```python
from build123d import *

# Parameters (mm, degrees)
SKETCH1_W                      = 50
SKETCH1_H                      = 100
SKETCH1_R                      = 15.2
SKETCH1_R_2                    = 2
BOSS_EXTRUDE1_DEPTH            = 33
CUT_EXTRUDE1_DEPTH             = 79.0320447
CHAMFER1_SIZE                  = 2.5
CUT_EXTRUDE2_DEPTH             = 68.029405
CUT_EXTRUDE4_DEPTH             = 39.051248
SKETCH6_W                      = 1.8
SKETCH6_H                      = 1.279654747
CUT_EXTRUDE5_DEPTH             = 79.03204487
FILLET1_R                      = 10
F_4_5_4_5_DIAMETER_HOLE1_D     = 4.5
F_4_5_4_5_DIAMETER_HOLE1_DEPTH = 8
F_4_5_4_5_DIAMETER_HOLE1_TIP   = 1.351936393


with BuildPart() as part:
    # Sketch1 → Boss-Extrude1 (new body)
    with BuildSketch(Plane(origin=(0, 0, 0), x_dir=(1, 0, 0), z_dir=(0, 1, 0))):
        Rectangle(SKETCH1_W, SKETCH1_H)
        with Locations(Location((0, 0, 0), (0, 0, 270))):
            Circle(SKETCH1_R, mode=Mode.SUBTRACT)
        with Locations(Location((0, 30.75, 0), (0, 0, 270))):
            Circle(SKETCH1_R_2, mode=Mode.SUBTRACT)
        with Locations(Location((0, -30.75, 0), (0, 0, 270))):
            Circle(SKETCH1_R_2, mode=Mode.SUBTRACT)
    extrude(amount=BOSS_EXTRUDE1_DEPTH)

    # Sketch2 → Cut-Extrude1 (cut, through all)
    with BuildSketch(Plane(origin=(25, 0, 0), x_dir=(0, 0, -1), z_dir=(1, 0, 0))):
        Polygon((50, 14), (12, 5), (-50, 33), (50, 33), align=None)
    extrude(amount=-CUT_EXTRUDE1_DEPTH, mode=Mode.SUBTRACT)

    # Chamfer1
    chamfer1_edges = [part.edges().sort_by_distance(p)[0] for p in [
        (0, 0, -32.75),
        (0, 0, 28.75),
    ]]
    chamfer(chamfer1_edges, length=CHAMFER1_SIZE)

    # Sketch3 → Cut-Extrude2 (cut)
    with BuildSketch(Plane(origin=(0, 24.345721694, 53.908383751), x_dir=(-1, 0, 0), z_dir=(0, -0.4115867224264983, -0.9113705996586748))):
        with BuildLine():
            Line((25, 9.495893667), (-25, 9.495893667))
            ThreePointArc((-25, 9.495893667), (0, 8.495893667), (25, 9.495893667))
        make_face()
    extrude(amount=CUT_EXTRUDE2_DEPTH, mode=Mode.SUBTRACT)

    # Sketch4 → Cut-Extrude4 (cut)
    with BuildSketch(Plane(origin=(0, 11.956721311, -50.483934426), x_dir=(-1, 0, 0), z_dir=(0, 0.23046638387921348, -0.9730802874900093))):
        with BuildLine():
            Line((25, 2.099804831), (-25, 2.099804831))
            ThreePointArc((-25, 2.099804831), (0, 1.099804831), (25, 2.099804831))
        make_face()
    extrude(amount=-CUT_EXTRUDE4_DEPTH, mode=Mode.SUBTRACT)

    # Sketch6 → Cut-Extrude5 (cut, through all)
    with BuildSketch(Plane.ZY.offset(25)):
        with Locations((-12.280764488, 4.639827374)):
            Rectangle(SKETCH6_W, SKETCH6_H)
    extrude(amount=-CUT_EXTRUDE5_DEPTH, mode=Mode.SUBTRACT)

    # Fillet1
    fillet1_edges = [part.edges().sort_by_distance(p)[0] for p in [
        (25, 16.5, 50),
        (25, 7, -50),
        (-25, 7, -50),
        (-25, 16.5, 50),
    ]]
    fillet(fillet1_edges, radius=FILLET1_R)

    # Ø4.5 (4.5) Diameter Hole1
    with Locations(Plane.XZ):
        with Locations((0, 42.5), (0, -42.5)):
            Hole(F_4_5_4_5_DIAMETER_HOLE1_D / 2, depth=F_4_5_4_5_DIAMETER_HOLE1_DEPTH)
            with Locations((0, 0, -(F_4_5_4_5_DIAMETER_HOLE1_DEPTH + F_4_5_4_5_DIAMETER_HOLE1_TIP / 2))):  # 118° drill point
                Cone(0, F_4_5_4_5_DIAMETER_HOLE1_D / 2, F_4_5_4_5_DIAMETER_HOLE1_TIP, mode=Mode.SUBTRACT)


solid = part.part
```
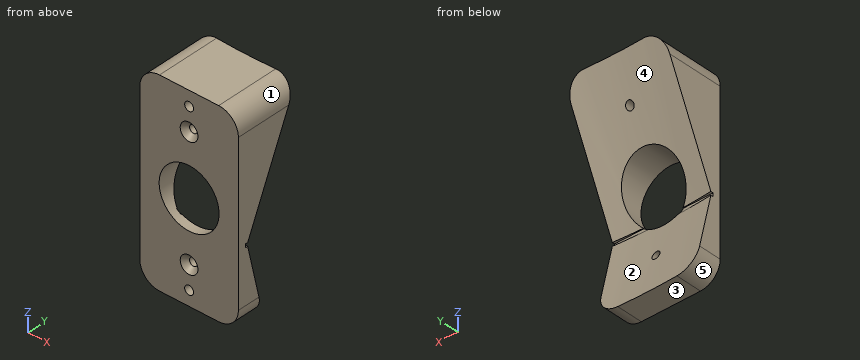
Work out the finished part from the listing and answer in its coordinate system (mm). Face numbers are marked on the shaded views. A direction names the side the tool comes from. Give positions to 0.01 mm unless a question says otherwise; leave off trailing zeros. Order: outer loops, then holes, each group sorted by start corner. A loop starts at its lowest first (then second) coordinate and runs counter-clockwise, first axis right, second up. Notation, with made-up numbers: (-3, -6.75) -> (52, -6.75) arc R27 ccw to (52, 28.25) -> close; hole circle Ø10 at (1, -15.75). An arc over 180 degrees is marked (long way). Answer as CSV lines item,"result". Start each with the question number.
(1) Each of these flat-tipped pins is pushed along its axis until it touches: pin 1 Ø1 at (x, y) = (19.5, 4.5) entering from -Z; pin 2 Ø0.9 at (x, z) = (13.5, -12.5) entering from +Y; pin 3 Ø10 at (x, z) = (12, 34) entering from +Y; pin 4 Ø10 at (x, y) = (-17, 5.5) entering from +Z. Where does it stop, or does it pass through?
(2) Consider line 1 along X through (y, z) = (6, 0); line 2 along X through (y, z) = (7, -30.5); line 3 along Z through (x, y) = (0, 2). Determine where each line is inside the solid, lowest interval first.
(3) For a pull along X with two mould halves and no side action, classify the marked faces 1, 2 and 3 as released by +X, released by -X, zero draft, split by the parting line, or undercut.
(4) Section A-A, the plane x = -17.5 is taken. Write down the section's boundary in (y, z).
(5) Which of the six approach directions +Z, -Z, +X, -X, +Y, -Y give full straight-line access (tool end or side, diameter ignored) to the marked faces 4 and 5?
Entries:
1,pin 1,"z = -49.17"
1,pin 2,"y = 4"
1,pin 3,"y = 27.2"
1,pin 4,"z = 50"
2,line 1,"-25 to -15.2, 15.2 to 25"
2,line 2,"-25 to -1.98, 1.98 to 25"
2,line 3,"-50 to -44.75, -40.25 to -33.25, -28.25 to -15.2, 15.2 to 28.25, 33.25 to 40.25, 44.75 to 50"
3,face 1,"released by +X"
3,face 2,"undercut"
3,face 3,"zero draft"
4,outline,"(0, -49.68) -> (13.4, -49.68) -> (4.76, -13.18) -> (4, -13.18) -> (4, -11.38) -> (4.72, -11.38) -> (32.3, 49.68) -> (0, 49.68) -> close"
5,face 4,"+Y"
5,face 5,"-Z, -X, +Y, -Y"
